Could you check a few things on this model? Use its own coordinates, in mm. Face numbers are marked on the shaded views. Coordinates: 2 decimals unless noted, no trailing zeros. Loops run counter-clockwise (first coordinate to the right, second up) from the corner with the lowest first, then second, coordinate; pieces in that order, holes last. Notation, with made-up numbers: (16.25, 83) -> (69.25, 83) arc R22 cw to (69.25, 111) -> close; hole circle Ø11 at (88.5, 45). An arc over 180 degrees is marked (long way). One line per question, with ' | ' between items.
```python
from build123d import *

# Parameters (mm, degrees)
SKETCH1_W           = 55.88
SKETCH1_H           = 26.1112
BOSS_EXTRUDE1_DEPTH = 8.89
SKETCH2_W           = 10.16
SKETCH2_H           = 3.869870213
SKETCH2_H_2         = 3.869870212
BOSS_EXTRUDE2_DEPTH = 1.27
SKETCH3_W           = 1.27
SKETCH3_H           = 3.869870213
BOSS_EXTRUDE3_DEPTH = 0.635


with BuildPart() as part:
    # Sketch1 → Boss-Extrude1 (new body)
    with BuildSketch(Plane.XY):
        with Locations((27.94, 13.0556)):
            Rectangle(SKETCH1_W, SKETCH1_H)
    extrude(amount=BOSS_EXTRUDE1_DEPTH)

    # Sketch2 → Boss-Extrude2 (add)
    with BuildSketch(Plane.XY.offset(8.89)):
        with Locations((5.08, 5.750232763)):
            Rectangle(SKETCH2_W, SKETCH2_H)
        with Locations((5.08, 13.0556)):
            Rectangle(SKETCH2_W, SKETCH2_H_2)
        with Locations((5.08, 20.360967237)):
            Rectangle(SKETCH2_W, SKETCH2_H)
        with Locations((50.8, 5.750232763)):
            Rectangle(SKETCH2_W, SKETCH2_H)
        with Locations((50.8, 20.360967237)):
            Rectangle(SKETCH2_W, SKETCH2_H)
    extrude(amount=BOSS_EXTRUDE2_DEPTH)

    # Sketch3 → Boss-Extrude3 (add)
    with BuildSketch(Plane(origin=(55.88, 0, 0), x_dir=(0, 0, -1), z_dir=(1, 0, 0))):
        with Locations((-9.525, 20.360967237)):
            Rectangle(SKETCH3_W, SKETCH3_H)
    extrude(amount=BOSS_EXTRUDE3_DEPTH)


solid = part.part
```
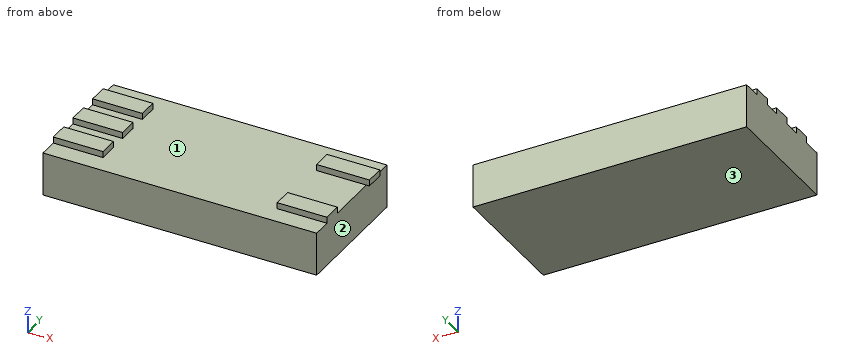
Q1. We'd pull the mould along X, two halves only. Please class the marked faces 1, 2 and 3: released by +X, released by -X, zero draft, split by the parting line, or undercut.
Values follow:
face 1: undercut | face 2: released by +X | face 3: zero draft
Q2. For pin 1 (1 mm diameter, centred on x = 53, z = 9.5, fed in from -Y); pin 2 (1 mm diameter, centred on x = 3.5, z = 10, fed in from +Y); pin 3 (3 mm diameter, centred on y = 13.5, z = 6.5, fed in from +X), each with a flat end and sliding along its axis, tell me the tip position at first contact or that it passes through.
Values follow:
pin 1: stops at y = 3.82 | pin 2: stops at y = 22.3 | pin 3: stops at x = 55.88
Q3. Imagine slicing it at A-A on y = 20.25. Write out the boundary of the cut face in (x, z) (3 decimals).
Values follow:
outline: (0, 0) -> (55.88, 0) -> (55.88, 8.89) -> (56.515, 8.89) -> (56.515, 10.16) -> (45.72, 10.16) -> (45.72, 8.89) -> (10.16, 8.89) -> (10.16, 10.16) -> (0, 10.16) -> close
Q4. Imagine slicing it at C-C on y = 5.5. Write out the boundary of the cut face in (x, z).
Values follow:
outline: (0, 0) -> (55.88, 0) -> (55.88, 10.16) -> (45.72, 10.16) -> (45.72, 8.89) -> (10.16, 8.89) -> (10.16, 10.16) -> (0, 10.16) -> close
Q5. Imagine slicing it at B-B on x = 28.5. Write out the boundary of the cut face in (y, z), plus the area to 3 significant figures.
Values follow:
outline: (0, 0) -> (26.11, 0) -> (26.11, 8.89) -> (0, 8.89) -> close | area: 232 mm2
Q6. Imagine slicing it at D-D on y = 16.75. Write out the boundary of the cut face in (x, z).
Values follow:
outline: (0, 0) -> (55.88, 0) -> (55.88, 8.89) -> (0, 8.89) -> close
Q7. Please list where these lines run through material, in increasing order: L1, parallel to X at y = 22.5, z = 8.75; L2, parallel to Z at x = 32.5, y = 6.25. Write a range as [from, to].
Values follow:
L1: x = [0, 55.88] | L2: z = [0, 8.89]
